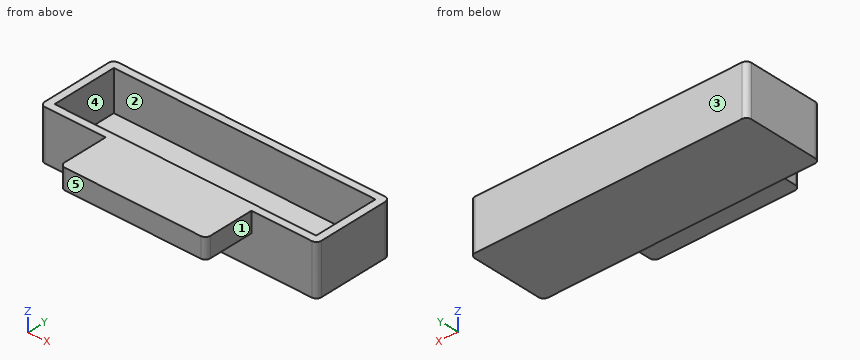
from build123d import *

# Parameters (mm, degrees)
F0_W     = 349.25
F0_H     = 101.6
F0_W_2   = 330.2
F0_H_2   = 82.55
F1_DEPTH = 63.5
F2_R     = 6.35
F3_W     = 330.2
F3_H     = 82.55
F4_DEPTH = 12.7
F5_W     = 184.15
F5_H     = 25.4
F6_DEPTH = 63.5
F7_R     = 6.35


with BuildPart() as f1:
    # F0 (on Top) → F1 (new body)
    with BuildSketch(Plane.XY):
        Rectangle(F0_W, F0_H)
        Rectangle(F0_W_2, F0_H_2, mode=Mode.SUBTRACT)
    extrude(amount=F1_DEPTH)

    # F2
    f2_edges = [f1.edges().sort_by_distance(p)[0] for p in [
        (-174.625, -50.8, 31.75),
        (174.625, -50.8, 31.75),
        (174.625, 50.8, 31.75),
        (-174.625, 50.8, 31.75),
    ]]
    fillet(f2_edges, radius=F2_R)

    # F3 (on Top) → F4 (join)
    with BuildSketch(Plane.XY):
        Rectangle(F3_W, F3_H)
    extrude(amount=F4_DEPTH)

    # F5 (on face) → F6 (join)
    with BuildSketch(Plane.XZ.offset(50.8)):
        with Locations((0, 50.8)):
            Rectangle(F5_W, F5_H)
    extrude(amount=F6_DEPTH)

    # F7
    f7_edges = [f1.edges().sort_by_distance(p)[0] for p in [
        (-92.075, -114.3, 50.8),
        (92.075, -114.3, 50.8),
    ]]
    fillet(f7_edges, radius=F7_R)


solid = f1.part
Check sheet for the modelled part. Datum: model origin and axes. Units: mm. Face numbers are marked on the shaded views. A direction names the side the tool comes from. Round coordinates to 2 decimals unless told otherwise and drop trailing zeros. Order: outer loops, then holes, each group sorted by start corner. A loop starts at its lowest first (then second) coordinate and runs counter-clockwise, first axis right, second up.
(1) Cross-section at A-A, the plane z = 43. Enter the section's corners in (x, y) (3 decimals).
(2) Access from +Z, -Z, +X, -X, +Y, -Y to the whole of each face (thin tool, end or side, straight path). Record for the marked faces 4 and 5.
(3) Cross-section at D-D, the plane z = 16. Enter the section's corners in (x, y) (3 decimals), and give its area (3 significant figures).
(4) Scan lines: probe 1 along Y at (x, z) = (19, 40) (3 decimals); probe 2 along Y at (x, z) = (-9.5, 30.5) (3 decimals); probe 3 along X at (y, z) = (-8.5, 30.5) (3 decimals). Record each from-to range of solid material in increasing order.
(5) Cross-section at C-C, the plane x = -82. Enter the section's corners in (y, z) (3 decimals), and give its area (3 significant figures).
(6) Go/stop test with flat-tipped pins: P1, Ø20.5, axis at y = -87.5, z = 52, coming from the +X side (3 decimals); P2, Ø20.5, axis at y = -67, z = 53, coming from the -X side (3 decimals); P3, Ø3, axis at x = -97.5, z = 6.5, coming from the -Y side; P4, Ø4, axis at y = -79, z = 36, coming from the -X side. Record where each tip stops, or that it passes through.
(7) Draft check along X on the marked faces 1, 2 and 3. Enter one of: pulls with the +X half, pulls with the -X half, needs draft (parallel to the pull), parting line crosses it, or undercut.
(8) Cross-section at B-B, the plane y = 22.5. Enter the section's corners in (x, z) (3 decimals).
Check sheet entries:
1. outline: (-174.625, -44.45) arc R6.35 ccw to (-168.275, -50.8) - (-92.075, -50.8) - (-92.075, -107.95) arc R6.35 ccw to (-85.725, -114.3) - (85.725, -114.3) arc R6.35 ccw to (92.075, -107.95) - (92.075, -50.8) - (168.275, -50.8) arc R6.35 ccw to (174.625, -44.45) - (174.625, 44.45) arc R6.35 ccw to (168.275, 50.8) - (-168.275, 50.8) arc R6.35 ccw to (-174.625, 44.45) - close; hole (-165.1, -41.275) - (165.1, -41.275) - (165.1, 41.275) - (-165.1, 41.275) - close
2. face 4: +Z
2. face 5: +Z, -Z, +X, -X, -Y
3. outline: (-174.625, -44.45) arc R6.35 ccw to (-168.275, -50.8) - (168.275, -50.8) arc R6.35 ccw to (174.625, -44.45) - (174.625, 44.45) arc R6.35 ccw to (168.275, 50.8) - (-168.275, 50.8) arc R6.35 ccw to (-174.625, 44.45) - close; hole (-165.1, -41.275) - (165.1, -41.275) - (165.1, 41.275) - (-165.1, 41.275) - close
3. area: 8,190 mm2
4. probe 1: y = -114.3 to -41.275, 41.275 to 50.8
4. probe 2: y = -50.8 to -41.275, 41.275 to 50.8
4. probe 3: x = -174.625 to -165.1, 165.1 to 174.625
5. outline: (-114.3, 38.1) - (-50.8, 38.1) - (-50.8, 0) - (50.8, 0) - (50.8, 63.5) - (41.275, 63.5) - (41.275, 12.7) - (-41.275, 12.7) - (-41.275, 63.5) - (-114.3, 63.5) - close
5. area: 3,870 mm2
6. P1: stops at x = 92.075
6. P2: stops at x = -92.075
6. P3: stops at y = -50.8
6. P4: passes through
7. face 1: pulls with the +X half
7. face 2: undercut
7. face 3: needs draft
8. outline: (-174.625, 0) - (174.625, 0) - (174.625, 63.5) - (165.1, 63.5) - (165.1, 12.7) - (-165.1, 12.7) - (-165.1, 63.5) - (-174.625, 63.5) - close
